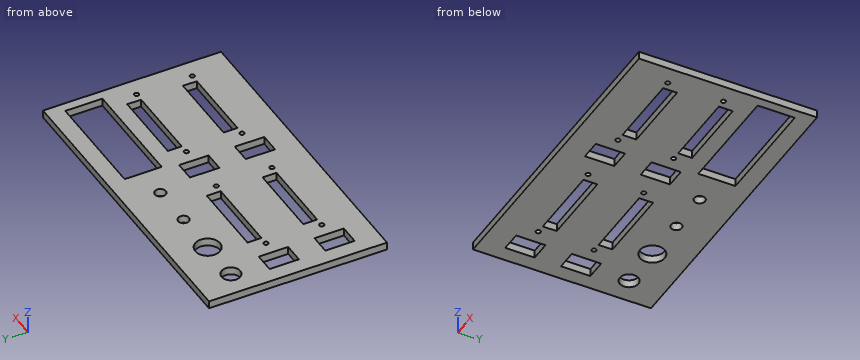
```python
from build123d import *

# Parameters (mm, degrees)
SKETCH1_W           = 200
SKETCH1_H           = 115
SKETCH1_R           = 1.5
SKETCH1_R_2         = 6
SKETCH1_R_3         = 8
SKETCH1_R_4         = 3.5
SKETCH1_W_2         = 49
SKETCH1_H_2         = 9
SKETCH1_W_3         = 13
SKETCH1_H_3         = 19
SKETCH1_W_4         = 71.5
SKETCH1_H_4         = 24
BOSS_EXTRUDE1_DEPTH = 5


with BuildPart() as part:
    # Sketch1 → Boss-Extrude1 (new body)
    with BuildSketch(Plane.XY):
        Rectangle(SKETCH1_W, SKETCH1_H)
        with Locations((-68, -32.5)):
            Circle(SKETCH1_R, mode=Mode.SUBTRACT)
        with Locations((-8, -32.5)):
            Circle(SKETCH1_R, mode=Mode.SUBTRACT)
        with Locations((87.971622358, -32.5)):
            Circle(SKETCH1_R, mode=Mode.SUBTRACT)
        with Locations((27.971622358, -32.5)):
            Circle(SKETCH1_R, mode=Mode.SUBTRACT)
        with Locations((87.971622358, 3.5)):
            Circle(SKETCH1_R, mode=Mode.SUBTRACT)
        with Locations((27.971622358, 3.5)):
            Circle(SKETCH1_R, mode=Mode.SUBTRACT)
        with Locations((-8, 3.5)):
            Circle(SKETCH1_R, mode=Mode.SUBTRACT)
        with Locations((-68, 3.5)):
            Circle(SKETCH1_R, mode=Mode.SUBTRACT)
        with Locations((-83.5, 34.5)):
            Circle(SKETCH1_R_2, mode=Mode.SUBTRACT)
        with Locations((-55.5, 34.5)):
            Circle(SKETCH1_R_3, mode=Mode.SUBTRACT)
        with Locations((1.5, 34.5)):
            Circle(SKETCH1_R_4, mode=Mode.SUBTRACT)
        with Locations((-26.5, 34.5)):
            Circle(SKETCH1_R_4, mode=Mode.SUBTRACT)
        with Locations((-38, -28)):
            Rectangle(SKETCH1_W_2, SKETCH1_H_2, mode=Mode.SUBTRACT)
        with Locations((-83.5, -32.5)):
            Rectangle(SKETCH1_W_3, SKETCH1_H_3, mode=Mode.SUBTRACT)
        with Locations((57.971622358, -28)):
            Rectangle(SKETCH1_W_2, SKETCH1_H_2, mode=Mode.SUBTRACT)
        with Locations((12.471622358, -32.5)):
            Rectangle(SKETCH1_W_3, SKETCH1_H_3, mode=Mode.SUBTRACT)
        with Locations((57.971622358, 8)):
            Rectangle(SKETCH1_W_2, SKETCH1_H_2, mode=Mode.SUBTRACT)
        with Locations((12.471622358, 3.5)):
            Rectangle(SKETCH1_W_3, SKETCH1_H_3, mode=Mode.SUBTRACT)
        with Locations((-38, 8)):
            Rectangle(SKETCH1_W_2, SKETCH1_H_2, mode=Mode.SUBTRACT)
        with Locations((-83.5, 3.5)):
            Rectangle(SKETCH1_W_3, SKETCH1_H_3, mode=Mode.SUBTRACT)
        with Locations((57.971622358, 34.5)):
            Rectangle(SKETCH1_W_4, SKETCH1_H_4, mode=Mode.SUBTRACT)
    extrude(amount=BOSS_EXTRUDE1_DEPTH)


solid = part.part
```
Part model, mm, in its own coordinate system. Round coordinates to 2 decimals unless told otherwise and drop trailing zeros. Write each loop counter-clockwise with the first axis right and the second up, starting at its lowest first coordinate (ties: lowest second). Pieces come first, ordered by that corner, then holes. Notation, with made-up numbers: M -39,-37 L 16,-37 A15 ccw 16,-19 Z; hole C -40,31.5 d11. An arc over 180 degrees is marked long. One line per question, with ' | ' between items.
(1) Probe line 1 along Y through (x, z) = (-37, 3.25); line 2 along Y through (x, z) = (76.5, 1.5); line 3 along X through (y, z) = (-40.5, 0.75). List the from-to ranges inside material, lowest first.
Answer key:
line 1: y = -57.5 to -32.5, -23.5 to 3.5, 12.5 to 57.5 | line 2: y = -57.5 to -32.5, -23.5 to 3.5, 12.5 to 22.5, 46.5 to 57.5 | line 3: x = -100 to -90, -77 to 5.97, 18.97 to 100
(2) Saw through at C-C on x = -26.5. Write the cut outline in (y, z).
Answer key:
outline: M -57.5,0 L -32.5,0 L -32.5,5 L -57.5,5 Z; M -23.5,0 L 3.5,0 L 3.5,5 L -23.5,5 Z; M 12.5,0 L 31,0 L 31,5 L 12.5,5 Z; M 38,0 L 57.5,0 L 57.5,5 L 38,5 Z
(3) Saw through at B-B on x = 58. Write the cut outline in (y, z).
Answer key:
outline: M -57.5,0 L -32.5,0 L -32.5,5 L -57.5,5 Z; M -23.5,0 L 3.5,0 L 3.5,5 L -23.5,5 Z; M 12.5,0 L 22.5,0 L 22.5,5 L 12.5,5 Z; M 46.5,0 L 57.5,0 L 57.5,5 L 46.5,5 Z
(4) Pin check, flat tip, straight feed: pin 1 (11 mm diameter, centred on x = -26.5, y = 34.5, fed in from +Z). Stop position of the tip, or through.
Answer key:
pin 1: stops at z = 5
(5) Saw through at D-D on z = 1.85. Count the separate pieces of the cut face and the enclosed holes in it, then the cut area to 3 significant figures.
Answer key:
separate pieces: 1 | enclosed holes: 21 | area: 18,100 mm^2
(6) Saw through at A-A on x = 1.5. Write the cut outline in (y, z), then the cut area to 3 significant figures.
Answer key:
outline: M -57.5,0 L 31,0 L 31,5 L -57.5,5 Z; M 38,0 L 57.5,0 L 57.5,5 L 38,5 Z | area: 540 mm^2
